from build123d import *

# Parameters (mm, degrees)
SKETCH1_W           = 71.12
SKETCH1_H           = 71.12
BOSS_EXTRUDE1_DEPTH = 43.18
SKETCH2_W           = 71.12
SKETCH2_H           = 71.12
SKETCH2_W_2         = 55.88
SKETCH2_H_2         = 55.88
CUT_EXTRUDE1_DEPTH  = 39.37
SKETCH4_W           = 50.8
SKETCH4_H           = 50.8
CUT_EXTRUDE2_DEPTH  = 35.56
CUT_EXTRUDE3_REACH  = 111.456
SKETCH5_R           = 1.651
SKETCH5_R_2         = 5.969
CUT_EXTRUDE4_REACH  = 111.456
SKETCH6_R           = 1.651
FILLET1_R           = 6.35
CUT_EXTRUDE5_REACH  = 106.665
CIRPATTERN1_COUNT   = 4
FILLET3_R           = 19.05
SKETCH8_R           = 3.175
CUT_EXTRUDE6_DEPTH  = 3.81


with BuildPart() as part:
    # Sketch1 → Boss-Extrude1 (new body)
    with BuildSketch(Plane.XY):
        with Locations((35.56, 35.56)):
            Rectangle(SKETCH1_W, SKETCH1_H)
    extrude(amount=BOSS_EXTRUDE1_DEPTH)

    # Sketch2 → Cut-Extrude1 (cut)
    with BuildSketch(Plane.XY.offset(43.18)):
        with Locations((35.56, 35.56)):
            Rectangle(SKETCH2_W, SKETCH2_H)
        with Locations((35.56, 35.56)):
            Rectangle(SKETCH2_W_2, SKETCH2_H_2, mode=Mode.SUBTRACT)
    extrude(amount=-CUT_EXTRUDE1_DEPTH, mode=Mode.SUBTRACT)

    # Sketch4 → Cut-Extrude2 (cut)
    with BuildSketch(Plane(origin=(0, 0, 0), x_dir=(-1, 0, 0), z_dir=(0, 0, -1))):
        with Locations((-35.56, 35.56)):
            Rectangle(SKETCH4_W, SKETCH4_H)
    extrude(amount=-CUT_EXTRUDE2_DEPTH, mode=Mode.SUBTRACT)

    # Sketch5 → Cut-Extrude3 (cut, up to next)
    with BuildSketch(Plane.XY.offset(43.18), mode=Mode.PRIVATE) as cut_extrude3_sk1:
        with Locations((35.56, 48.006)):
            Circle(SKETCH5_R)
    cut_extrude3_tool1 = extrude(cut_extrude3_sk1.sketch, amount=-CUT_EXTRUDE3_REACH, mode=Mode.PRIVATE) & part.part
    # Sketch5 → Cut-Extrude3 (cut, up to next)
    with BuildSketch(Plane.XY.offset(43.18), mode=Mode.PRIVATE) as cut_extrude3_sk2:
        with Locations((48.006, 35.56)):
            Circle(SKETCH5_R)
    cut_extrude3_tool2 = extrude(cut_extrude3_sk2.sketch, amount=-CUT_EXTRUDE3_REACH, mode=Mode.PRIVATE) & part.part
    # Sketch5 → Cut-Extrude3 (cut, up to next)
    with BuildSketch(Plane.XY.offset(43.18), mode=Mode.PRIVATE) as cut_extrude3_sk3:
        with Locations((35.56, 23.114)):
            Circle(SKETCH5_R)
    cut_extrude3_tool3 = extrude(cut_extrude3_sk3.sketch, amount=-CUT_EXTRUDE3_REACH, mode=Mode.PRIVATE) & part.part
    # Sketch5 → Cut-Extrude3 (cut, up to next)
    with BuildSketch(Plane.XY.offset(43.18), mode=Mode.PRIVATE) as cut_extrude3_sk4:
        with Locations((23.114, 35.56)):
            Circle(SKETCH5_R)
    cut_extrude3_tool4 = extrude(cut_extrude3_sk4.sketch, amount=-CUT_EXTRUDE3_REACH, mode=Mode.PRIVATE) & part.part
    # Sketch5 → Cut-Extrude3 (cut, up to next)
    with BuildSketch(Plane.XY.offset(43.18), mode=Mode.PRIVATE) as cut_extrude3_sk5:
        with Locations((35.56, 35.56)):
            Circle(SKETCH5_R_2)
    cut_extrude3_tool5 = extrude(cut_extrude3_sk5.sketch, amount=-CUT_EXTRUDE3_REACH, mode=Mode.PRIVATE) & part.part
    add(cut_extrude3_tool1.solids().sort_by_distance((35.56, 48.006, 43.18))[0], mode=Mode.SUBTRACT)
    add(cut_extrude3_tool2.solids().sort_by_distance((48.006, 35.56, 43.18))[0], mode=Mode.SUBTRACT)
    add(cut_extrude3_tool3.solids().sort_by_distance((35.56, 23.114, 43.18))[0], mode=Mode.SUBTRACT)
    add(cut_extrude3_tool4.solids().sort_by_distance((23.114, 35.56, 43.18))[0], mode=Mode.SUBTRACT)
    add(cut_extrude3_tool5.solids().sort_by_distance((35.56, 35.56, 43.18))[0], mode=Mode.SUBTRACT)

    # Sketch6 → Cut-Extrude4 (cut, up to next)
    with BuildSketch(Plane(origin=(0, 0, 0), x_dir=(-1, 0, 0), z_dir=(0, 0, -1)), mode=Mode.PRIVATE) as cut_extrude4_sk1:
        with Locations((-35.56, 67.31)):
            Circle(SKETCH6_R)
    cut_extrude4_tool1 = extrude(cut_extrude4_sk1.sketch, amount=-CUT_EXTRUDE4_REACH, mode=Mode.PRIVATE) & part.part
    # Sketch6 → Cut-Extrude4 (cut, up to next)
    with BuildSketch(Plane(origin=(0, 0, 0), x_dir=(-1, 0, 0), z_dir=(0, 0, -1)), mode=Mode.PRIVATE) as cut_extrude4_sk2:
        with Locations((-3.81, 35.56)):
            Circle(SKETCH6_R)
    cut_extrude4_tool2 = extrude(cut_extrude4_sk2.sketch, amount=-CUT_EXTRUDE4_REACH, mode=Mode.PRIVATE) & part.part
    # Sketch6 → Cut-Extrude4 (cut, up to next)
    with BuildSketch(Plane(origin=(0, 0, 0), x_dir=(-1, 0, 0), z_dir=(0, 0, -1)), mode=Mode.PRIVATE) as cut_extrude4_sk3:
        with Locations((-35.56, 3.81)):
            Circle(SKETCH6_R)
    cut_extrude4_tool3 = extrude(cut_extrude4_sk3.sketch, amount=-CUT_EXTRUDE4_REACH, mode=Mode.PRIVATE) & part.part
    # Sketch6 → Cut-Extrude4 (cut, up to next)
    with BuildSketch(Plane(origin=(0, 0, 0), x_dir=(-1, 0, 0), z_dir=(0, 0, -1)), mode=Mode.PRIVATE) as cut_extrude4_sk4:
        with Locations((-67.31, 35.56)):
            Circle(SKETCH6_R)
    cut_extrude4_tool4 = extrude(cut_extrude4_sk4.sketch, amount=-CUT_EXTRUDE4_REACH, mode=Mode.PRIVATE) & part.part
    add(cut_extrude4_tool1.solids().sort_by_distance((35.56, 67.31, 0))[0], mode=Mode.SUBTRACT)
    add(cut_extrude4_tool2.solids().sort_by_distance((3.81, 35.56, 0))[0], mode=Mode.SUBTRACT)
    add(cut_extrude4_tool3.solids().sort_by_distance((35.56, 3.81, 0))[0], mode=Mode.SUBTRACT)
    add(cut_extrude4_tool4.solids().sort_by_distance((67.31, 35.56, 0))[0], mode=Mode.SUBTRACT)

    # Fillet1
    fillet1_edges = [part.edges().sort_by_distance(p)[0] for p in [
        (60.96, 10.16, 17.78),
        (60.96, 60.96, 17.78),
        (10.16, 60.96, 17.78),
        (10.16, 10.16, 17.78),
    ]]
    fillet(fillet1_edges, radius=FILLET1_R)

    # Sketch7 → Cut-Extrude5 (cut, up to next)
    with BuildSketch(Plane.ZY.offset(-7.62), mode=Mode.PRIVATE) as cut_extrude5_sk1:
        with BuildLine():
            Line((10.16, 20.32), (10.16, 50.8))
            ThreePointArc((10.16, 50.8), (12.019871939, 55.290128061), (16.51, 57.15))
            Line((16.51, 57.15), (29.21, 57.15))
            ThreePointArc((29.21, 57.15), (33.700128061, 55.290128061), (35.56, 50.8))
            Line((35.56, 50.8), (35.56, 20.32))
            ThreePointArc((35.56, 20.32), (33.700128061, 15.829871939), (29.21, 13.97))
            Line((29.21, 13.97), (16.51, 13.97))
            ThreePointArc((16.51, 13.97), (12.019871939, 15.829871939), (10.16, 20.32))
        make_face()
    cut_extrude5_tool1 = extrude(cut_extrude5_sk1.sketch, amount=-CUT_EXTRUDE5_REACH, mode=Mode.PRIVATE) & part.part
    cut_extrude5 = cut_extrude5_tool1.solids().sort_by_distance((7.62, 35.56, 22.86))[0]
    add(cut_extrude5, mode=Mode.SUBTRACT)

    # CirPattern1: Cut-Extrude5 ×4 about axis
    cirpattern1_axis = Axis((35.56, 35.56, 0), (0, 0, 1))
    for i in range(1, CIRPATTERN1_COUNT):
        add(cut_extrude5.rotate(cirpattern1_axis, i * 360 / CIRPATTERN1_COUNT), mode=Mode.SUBTRACT)

    # Fillet3
    fillet3_edges = [part.edges().sort_by_distance(p)[0] for p in [
        (0, 0, 1.905),
        (0, 71.12, 1.905),
        (71.12, 71.12, 1.905),
        (71.12, 0, 1.905),
    ]]
    fillet(fillet3_edges, radius=FILLET3_R)

    # Sketch8 → Cut-Extrude6 (cut)
    with BuildSketch(Plane(origin=(0, 0, 35.56), x_dir=(-1, 0, 0), z_dir=(0, 0, -1))):
        with Locations((-35.56, 48.006)):
            Circle(SKETCH8_R)
        with Locations((-23.114, 35.56)):
            Circle(SKETCH8_R)
        with Locations((-35.56, 23.114)):
            Circle(SKETCH8_R)
        with Locations((-48.006, 35.56)):
            Circle(SKETCH8_R)
    extrude(amount=-CUT_EXTRUDE6_DEPTH, mode=Mode.SUBTRACT)


solid = part.part
The model under review builds one solid part; all positions refer to its coordinate system, in mm. A direction names the side the tool comes from. Coordinates: 2 decimals unless noted, no trailing zeros. Write each loop counter-clockwise with the first axis right and the second up, starting at its lowest first coordinate (ties: lowest second). Pieces come first, ordered by that corner, then holes. Notation, with made-up numbers: (84.25, 65) - (126.25, 65) arc R29 cw to (126.25, 93) - close; hole circle Ø4 at (78.5, -11.5). An arc over 180 degrees is marked (long way). Answer as a JSON object with one key per item and string values. Group by question number.
1. Add section C-C (z = 27). Give the boundary of the cut face in (x, y).
2. Mouldability with a two-part tool opening along Z and no side actions: class faces 1 (the face through (65.39, 65.69, 1.93)), 2 (the face through (9, 57.15, 23)), 3 (the face through (34, 47, 39.37)) as pulls with the +Z half, pulls with the -Z half, needs draft (parallel to the pull), parting line crosses it, or undercut.
3. Add section D-D (y = 53.5). Give the boundary of the cut face in (x, z), plus the area to 3 significant figures.
4. Clearance check with flat-ended pins moving along their axes: pin 1 Ø8 at (x, y) = (11, 31) entering from -Z; pin 2 Ø3 at (x, y) = (49.5, 36.5) entering from -Z; pin 3 Ø4.5 at (x, y) = (3.81, 35.56) entering from +Z; pin 4 Ø5 at (x, z) = (14, 33) entering from -Y. State where each tip first meets the part, or that it passes through.
5. Machinability: for faces 4 (the face through (59.1, 59.1, 18)), 5 (the face through (61.99, 55.34, 12.07)), 6 (the face through (36, 9, 10.16)), which of the approach directions +Z, -Z, +X, -X, +Y, -Y give a long, thin tool a straight path to every point of the face, cutting with its end or side? Answer none if there is none.
6. To check wall thickness, follow probe 1 along Y at (x, z) = (35.56, 41) (3 decimals); probe 2 along Y at (x, z) = (35, 37); probe 3 along X at (y, z) = (34.5, 36). State the ranges of each line that lie inside material, in increasing order.
7. Add section A-A (y = 3.81). Give the boundary of the cut face in (x, z), plus the area to 3 significant figures.
Findings:
{
 "1": {"outline": "(7.62, 7.62) - (13.97, 7.62) - (13.97, 10.69) arc R6.35 cw to (10.69, 13.97) - (7.62, 13.97) - close; (7.62, 57.15) - (10.69, 57.15) arc R6.35 cw to (13.97, 60.43) - (13.97, 63.5) - (7.62, 63.5) - close; (57.15, 7.62) - (63.5, 7.62) - (63.5, 13.97) - (60.43, 13.97) arc R6.35 cw to (57.15, 10.69) - close; (57.15, 60.43) arc R6.35 cw to (60.43, 57.15) - (63.5, 57.15) - (63.5, 63.5) - (57.15, 63.5) - close"},
 "2": {"face 1": "needs draft", "face 2": "undercut", "face 3": "pulls with the -Z half"},
 "3": {"outline": "(0.05, 0) - (10.16, 0) - (10.16, 10.76) - (7.62, 10.76) - (7.62, 3.81) - (0.05, 3.81) - close; (7.62, 34.96) - (10.16, 34.96) - (10.16, 35.56) - (60.96, 35.56) - (60.96, 34.96) - (63.5, 34.96) - (63.5, 43.18) - (7.62, 43.18) - close; (60.96, 0) - (71.07, 0) - (71.07, 3.81) - (63.5, 3.81) - (63.5, 10.76) - (60.96, 10.76) - close", "area": "541 mm²"},
 "4": {"pin 1": "z = 0", "pin 2": "z = 35.56", "pin 3": "z = 3.81", "pin 4": "y = 7.62"},
 "5": {"face 4": "-Z", "face 5": "+X, -X", "face 6": "+Y, -Y"},
 "6": {"probe 1": "7.62 to 21.463, 24.765 to 29.591, 41.529 to 46.355, 49.657 to 63.5", "probe 2": "7.62 to 19.99, 26.24 to 29.62, 41.5 to 44.88, 51.13 to 63.5", "probe 3": "7.62 to 20.12, 26.11 to 29.69, 41.43 to 45.01, 51 to 63.5"},
 "7": {"outline": "(7.62, 0) - (33.91, 0) - (33.91, 3.81) - (7.62, 3.81) - close; (37.21, 0) - (63.5, 0) - (63.5, 3.81) - (37.21, 3.81) - close", "area": "200 mm²"}
}
